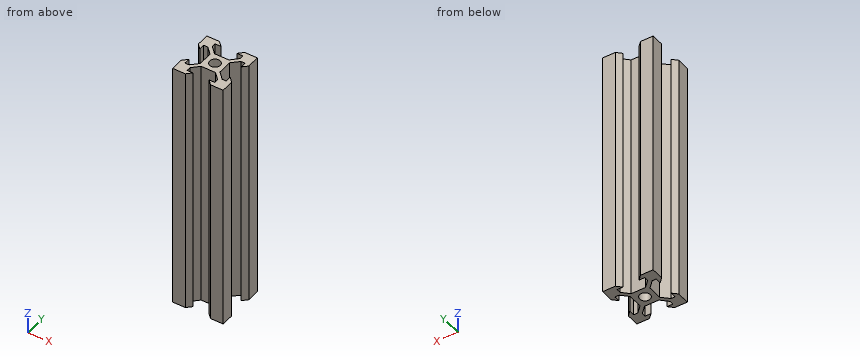
```python
from build123d import *

# Parameters (mm, degrees)
SKETCH1_R           = 2.1
BOSS_EXTRUDE1_DEPTH = 100


with BuildPart() as part:
    # Sketch1 → Boss-Extrude1 (new body)
    with BuildSketch(Plane.XY):
        Polygon((-10, 10), (-10, 5), (-8.2, 3.2), (-8.2, 5.499339828), (-6.56, 5.499339828), (-3.900660172, 2.84), (-3.900660172, -2.84), (-6.56, -5.499339828), (-8.2, -5.499339828), (-8.2, -3.2), (-10, -5), (-10, -10), (-5, -10), (-3.2, -8.2), (-5.499339828, -8.2), (-5.499339828, -6.56), (-2.84, -3.900660172), (2.84, -3.900660172), (5.499339828, -6.56), (5.499339828, -8.2), (3.2, -8.2), (5, -10), (10, -10), (10, -5), (8.2, -3.2), (8.2, -5.499339828), (6.56, -5.499339828), (3.900660172, -2.84), (3.900660172, 2.84), (6.56, 5.499339828), (8.2, 5.499339828), (8.2, 3.2), (10, 5), (10, 10), (5, 10), (3.2, 8.2), (5.499339828, 8.2), (5.499339828, 6.56), (2.84, 3.900660172), (-2.84, 3.900660172), (-5.499339828, 6.56), (-5.499339828, 8.2), (-3.2, 8.2), (-5, 10), align=None)
        Circle(SKETCH1_R, mode=Mode.SUBTRACT)
    extrude(amount=-BOSS_EXTRUDE1_DEPTH)


solid = part.part
```
Geometry: final body of the model. Coordinates: model frame, mm. Coordinates: 2 decimals unless noted, no trailing zeros. Order: outer loops, then holes, each group sorted by start corner. A loop starts at its lowest first (then second) coordinate and runs counter-clockwise, first axis right, second up.
Item 1: Contact query for flat-ended pins moving along their axis: P1, Ø1.1, axis at y = -4, z = -56, coming from the -X side; P2, Ø3.5, axis at x = 0, y = 0, coming from the +Z side; P3, Ø1, axis at y = 0, z = -19.5, coming from the -X side; P4, Ø4.5, axis at y = -1.5, z = -40, coming from the +X side. Output: stop coordinate, or through.
Answer:
P1: stops at x = -9.55
P2: passes through
P3: stops at x = -3.9
P4: stops at x = 8.75
Item 2: Section query A-A (y = 0). Output: boundary loops of the cut face in (x, z).
Answer:
outline: (-3.9, -100) - (-2.1, -100) - (-2.1, 0) - (-3.9, 0) - close; (2.1, -100) - (3.9, -100) - (3.9, 0) - (2.1, 0) - close
Item 3: Material intervals for line 1 along Y through (x, z) = (0, -28.5); line 2 along X through (y, z) = (0.25, -44); line 3 along Y through (x, z) = (4.5, -60), sorted ascending.
Answer:
line 1: y = -3.9 to -2.1, 2.1 to 3.9
line 2: x = -3.9 to -2.09, 2.09 to 3.9
line 3: y = -9.5 to -8.2, -5.56 to -3.44, 3.44 to 5.56, 8.2 to 9.5
